Autodesk Inventor part; units mm, degrees
ref_plane "Work Plane1" through (29, 0, 0) normal (0, -1, 0) x (1, 0, 0)
ref_plane "YZ Plane" through (0, 0, 0) normal (1, 0, 0) x (0, 1, 0)
ref_plane "XZ Plane" through (0, 0, 0) normal (0, 1, 0) x (-1, 0, 0)
sketch "Sketch1" plane through (0, 0, 0) normal (0, 0, 1) x (1, 0, 0)
  line L0 (0.2879, 0) -> (25.4, 0)
  line L1 (25.4, 0) -> (25.4, 2.413)
  line L2 (25.4, 2.413) -> (1.5878, 2.413)
  line L3 (1.5878, 2.413) -> (0.0002, 2.413)
  line L4 (0.0002, 2.413) -> (0, 2.413)
  line L5 (0, 2.413) -> (0, 4.5847)
  line L6 (0, 4.5847) -> (-2.5654, 4.5847)
  line L7 (-2.5654, 4.5847) -> (-2.5654, 1.8624)
  line L8 (-2.5654, 1.8624) -> (-0.7874, 1.8624)
  line L9 (-0.7874, 1.8624) -> (0.2879, 0)
  line L10 (-8.1585, 0) -> (30.9931, 0)
  line L11 (0, -0.9169) -> (0, 5.5016)
  line L12 (1.5878, 2.413) -> (0, 2.413) construction
  dimension "d1" = 23.8122
  dimension "d2" = 1.5876
  dimension "d3" = 2.5654
  dimension "d4" = 1.778
  dimension "d5" = 60
  dimension "d6" = 4.826
  dimension "d7" = 4.826
  dimension "d8" = 3.7248
  dimension "d9" = 9.1694
  dimension "d26" = 25.4
revolve "Body" add sketch "Sketch1" angle 360 about axis through (0.2879, 0, 0) along (1, 0, 0) contours L9 L11 L3 L2 L1 L0 | L9 L8 L7 L6 L5 L11
sketch "Sketch2" plane through (-2.5654, 0, 0) normal (-1, 0, 0) x (0, 0, 1)
  circle A0 centre (0, 0) radius 1.8624
  line L0 (0, -6.4186) -> (0, 6.4186)
  line L1 (-6.4186, 0) -> (6.4186, 0)
  line L2 (1.8624, 0) -> (0.9312, -1.6129)
  line L3 (0.9312, -1.6129) -> (-0.9312, -1.6129)
  line L4 (-0.9312, -1.6129) -> (-1.8624, 0)
  line L5 (-1.8624, 0) -> (-0.9312, 1.6129)
  line L6 (-0.9312, 1.6129) -> (0.9312, 1.6129)
  line L7 (0.9312, 1.6129) -> (1.8624, 0)
extrude "Slot" add sketch "Sketch2" against normal up to next contours L7 A0 | A0 L2 | L6 L0 A0 | A0 L0 L3 | L0 L6 A0 | A0 L3 L0 | L4 A0 | A0 L5
fillet "Fillet1" radius 1.778 1 edges at (-2.5654, -4.5847, 0)
thread "Thread"
chamfer "Chamfer1" distance 0.4869 distance2 0.4869 1 edges at (25.4, -2.413, 0) measured on face at (25.4, 0.9527, 0.2826)
ref_plane "Work Plane1" through (29, 0, 0) normal (0, -1, 0) x (1, 0, 0)
fillet "Fillet2" radius 0.1 1 edges at (0.0002, -2.413, 0)
equation "\"d30\" = R"
equation "\"d17\" = RR"
equation "\"d13\" = GEL"
equation "\"d15\" = -0.5 * SPD + 0.5 * GD"
equation "\"d16\" = GUL"
equation "\"d1\" = GEL"
equation "\"d3\" = KOH"
equation "\"d4\" = INTI"
equation "\"d6\" = GD"
equation "\"d7\" = BDM"
equation "\"d8\" = 1.1547 * SW"
equation "\"d9\" = KOD"
equation "\"d26\" = NLG"
equation "\"GD\" = NND"
equation "\"NLG\" = 25.4"
equation "\"GEL\" = 23.81225"
equation "\"KOD\" = 9.1694"
equation "\"KOH\" = 2.5654"
equation "\"INTI\" = 1.778"
equation "\"GAL\" = 1.5875"
equation "\"GUL\" = 0.48692"
equation "\"BDM\" = NND"
equation "\"SW\" = 3.2258"
equation "\"RR\" = 1.778"
equation "\"SPD\" = GD1"
equation "\"R\" = 0.1"
equation "\"KR\" = 4.699"
equation "\"GD1\" = 3.85216"
equation "\"THREADDIA\" = 4.826"
equation "\"FAWI\" = 45deg"
equation "\"KOH1\" = 1.778"
equation "\"NND\" = 4.826"
equation "\"TOA\" = 30deg"
equation "\"E0\" = 1.155 * SW"
properties part number "Unbrako - 10 x 1" material "Steel, Mild"
Read the model definition and answer for the solid it produces. Units are mm, in the model's axes. A direction names the side the tool comes from. Give positions to 0.01 mm unless a question says otherwise; leave off trailing zeros. Loops run counter-clockwise (first coordinate to the right, second up) from the corner with the lowest first, then second, coordinate; pieces in that order, holes last. Notation, with made-up numbers: M 43,-24 L 54,-24 A14 ccw 54,-16 Z; hole C 61,-32.75 d4. An arc over 180 degrees is marked long. Write each question's results on one line, items separated by ' | '.
1. The mould has two halves that part along Z. Classify faces 1 (the face through (-2.565, -2, 0)), 2 (the face through (-1.6, -0.8, 1.4)), 3 (the face through (-0.4, -3.64, 2.79)): pulls with the +Z half, pulls with the -Z half, needs draft (parallel to the pull), parting line crosses it, or undercut.
Values:
face 1: needs draft | face 2: undercut | face 3: parting line crosses it
2. Straight lines are drawn through the part: line 1 (X direction, y = -1, z = -2.5); line 2 (Z direction, x = 22.25, y = 2); line 3 (Y direction, x = 24, z = -0.25). For each, find the intervals that lie inside material, in ascending order. Write a range as [from, to].
Values:
line 1: x = [-2.57, 0] | line 2: z = [-1.35, 1.35] | line 3: y = [-2.4, 2.4]
3. Section A-A on x = 15.75 is taken. Give the vertices of the cut face in (y, z), plus the area to 3 significant figures.
Values:
outline: C 0,0 d4.83 | area: 18.3 mm^2
4. A tool of negligible diameter and unlimited length cuts with its end or side. For faces 4 (the face through (25.4, 0, 0)), 5 (the face through (-2, -1.613, 0)), 6 (the face through (0, 3, -1)), from which of +Z, -Z, +X, -X, +Y, -Y can it reach the whole face along a straight path? Write none if from no direction.
Values:
face 4: +Z, -Z, +X, +Y, -Y | face 5: -X | face 6: +X
5. Given pin 1 (4 mm diameter, centred on x = 21, y = 1, fed in from +Z); pin 2 (0.6 mm diameter, centred on x = -1.5, z = 0.5, fed in from +Y); pin 3 (1 mm diameter, centred on y = -3.5, z = -1.5, fed in from +X), each flat-ended and moving along its own axis, determine where each tip first touches the part or whether it passes through.
Values:
pin 1: stops at z = 2.41 | pin 2: stops at y = 4.51 | pin 3: stops at x = 0
